Part model, mm, in its own coordinate system. A direction names the side the tool comes from. Round coordinates to 2 decimals unless told otherwise and drop trailing zeros. Write each loop counter-clockwise with the first axis right and the second up, starting at its lowest first coordinate (ties: lowest second). Pieces come first, ordered by that corner, then holes. Notation, with made-up numbers: M -7.5,-5.5 L 25.5,-5.5 A18 ccw 25.5,14.5 Z; hole C 36,40.25 d5. An arc over 180 degrees is marked long. One line per question, with ' | ' between items. Start each with the question number.
1) Wall check: probe 1 along Y at (x, z) = (-1, 2.75) (3 decimals); probe 2 along X at (y, z) = (2.5, 1); probe 3 along X at (y, z) = (3, 1.25). Give the ranges that are in metal, low to high. Write a range as [from, to].
2) Saw through at B-B (y = 5). List the corners of the cut face in (x, z) (3 decimals), plus the area to 3 significant figures.
3) Saw through at A-A (x = 0). List the corners of the cut face in (y, z) (3 decimals).
4) Drop flat-ended pins along their axis: pin 1 Ø1 at (x, z) = (-2.5, -2) entering from +Y (3 decimals); pin 2 Ø2.5 at (y, z) = (4.5, 1.5) entering from -X; pin 3 Ø3 at (x, y) = (2, 7.5) entering from +Z; pin 4 Ø1.8 at (y, z) = (5, -2) entering from -X. Give the stop position or say it passes through.
5) Saw through at C-C (z = 0). List the corners of the cut face in (x, y) (3 decimals).
6) Mould opens along X. For faces 3 (the face through (-1.29, 4.7, -0.41)), 4 (the face through (0.7, 0, -1.4)), 5 (the face through (2.8, 4.7, -1.5)) say: pulls with the +X half, pulls with the -X half, needs draft (parallel to the pull), parting line crosses it, or undercut.
7) Saw through at D-D (z = 2.5). List the corners of the cut face in (x, y) (3 decimals).
8) Tool access for faces 1 (the face through (-1.191, 5, 2)), 2 (the face through (0.7, 9.525, -1.4)): list every direction of +Z, -Z, +X, -X, +Y, -Y with a clear straight run to the whole face (end or side of a thin tool).
```python
from build123d import *

# Parameters (mm, degrees)
SKETCH1_R                 = 3.175
BOSS_EXTRUDE1_DEPTH       = 9.525
TAP_DRILL_FOR_6_32_TAP1_D = 2.7051
CUT_EXTRUDE1_DEPTH        = 11.530283709
CUT_EXTRUDE1_DEPTH_BACK   = 11.530283709


with BuildPart() as part:
    # Sketch1 → Boss-Extrude1 (new body)
    with BuildSketch(Plane(origin=(0, 0, 0), x_dir=(1, 0, 0), z_dir=(0, 1, 0))):
        with Locations(Location((0, 0, 0), (0, 0, 90))):
            Circle(SKETCH1_R)
    extrude(amount=BOSS_EXTRUDE1_DEPTH)

    # Tap Drill for #6-32 Tap1 (through all)
    with Locations(Plane(origin=(0, 9.525, 0), x_dir=(1, 0, 0), z_dir=(0, 1, 0))):
        with Locations((0, 0)):
            Hole(TAP_DRILL_FOR_6_32_TAP1_D / 2)

    # Sketch4 → Cut-Extrude1 (cut, two sides: drawn at the far end of the back side and taken through both)
    with BuildSketch(Plane.XY.offset(-CUT_EXTRUDE1_DEPTH_BACK)):
        with BuildLine():
            Line((1.190625, 6.35), (1.190625, 3.175))
            ThreePointArc((1.190625, 3.175), (0, 1.984375), (-1.190625, 3.175))
            Line((-1.190625, 3.175), (-1.190625, 6.35))
            ThreePointArc((-1.190625, 6.35), (0, 7.540625), (1.190625, 6.35))
        make_face()
    extrude(amount=CUT_EXTRUDE1_DEPTH + CUT_EXTRUDE1_DEPTH_BACK, mode=Mode.SUBTRACT)


solid = part.part
```
Answer key:
1) probe 1: y = [0, 2.529], [6.996, 9.525] | probe 2: x = [-3.01, -0.98], [0.98, 3.01] | probe 3: x = [-2.92, -1.18], [1.18, 2.92]
2) outline: M -1.191,-2.943 L -1.191,-0.642 A1.353 cw -1.191,0.642 L -1.191,2.943 A3.175 ccw Z; M 1.191,-2.943 A3.175 ccw 1.191,2.943 L 1.191,0.642 A1.353 cw 1.191,-0.642 Z | area: 16.6 mm2
3) outline: M 0,-3.175 L 1.984,-3.175 L 1.984,-1.353 L 0,-1.353 Z; M 0,1.353 L 1.984,1.353 L 1.984,3.175 L 0,3.175 Z; M 7.541,-3.175 L 9.525,-3.175 L 9.525,-1.353 L 7.541,-1.353 Z; M 7.541,1.353 L 9.525,1.353 L 9.525,3.175 L 7.541,3.175 Z
4) pin 1: stops at y = 9.525 | pin 2: stops at x = -3.17 | pin 3: stops at z = 3.14 | pin 4: stops at x = -2.98
5) outline: M -3.175,0 L -1.353,0 L -1.353,9.525 L -3.175,9.525 Z; M 1.353,0 L 3.175,0 L 3.175,9.525 L 1.353,9.525 Z
6) face 3: undercut | face 4: needs draft | face 5: parting line crosses it
7) outline: M -1.957,0 L 1.957,0 L 1.957,9.525 L -1.957,9.525 Z; hole M -1.191,3.175 A1.191 ccw 1.191,3.175 L 1.191,6.35 A1.191 ccw -1.191,6.35 Z
8) face 1: +Z, -Z | face 2: +Z, -Z, +X, -X, +Y
